Build history of the part. All positions in model axes, mm. Face numbers are marked on the shaded views. A direction names the side the tool comes from. Round coordinates to 2 decimals unless told otherwise and drop trailing zeros. Write each loop counter-clockwise with the first axis right and the second up, starting at its lowest first coordinate (ties: lowest second). Pieces come first, ordered by that corner, then holes. Notation, with made-up numbers: (-36, -4.75) -> (-11, -4.75) arc R32 cw to (-11, 22.25) -> close; hole circle Ø10 at (42.25, 78). An arc over 180 degrees is marked (long way). Answer in a Markdown table with one row per item. Add a question column.
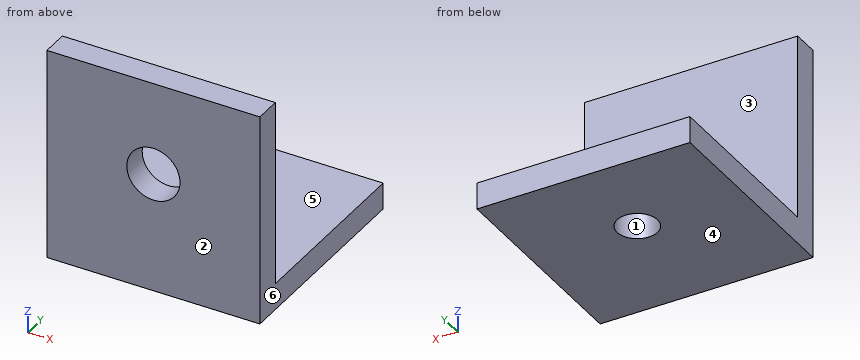
from build123d import *

# Parameters (mm, degrees)
SKETCH1_W           = 25.4
SKETCH1_H           = 25.4
BOSS_EXTRUDE1_DEPTH = 3.175
SKETCH6_W           = 25.4
SKETCH6_H           = 3.175
BOSS_EXTRUDE2_DEPTH = 22.225
SKETCH8_R           = 2.413
CUT_EXTRUDE3_DEPTH  = 3.175
SKETCH9_R           = 3.175
CUT_EXTRUDE4_DEPTH  = 3.175


with BuildPart() as part:
    # Sketch1 → Boss-Extrude1 (new body)
    with BuildSketch(Plane(origin=(0, 0, 0), x_dir=(1, 0, 0), z_dir=(0, 1, 0))):
        Rectangle(SKETCH1_W, SKETCH1_H)
    extrude(amount=BOSS_EXTRUDE1_DEPTH)

    # Sketch6 → Boss-Extrude2 (add)
    with BuildSketch(Plane(origin=(0, 3.175, 0), x_dir=(1, 0, 0), z_dir=(0, 1, 0))):
        with Locations((0, 11.1125)):
            Rectangle(SKETCH6_W, SKETCH6_H)
    extrude(amount=BOSS_EXTRUDE2_DEPTH)

    # Sketch8 → Cut-Extrude3 (cut)
    with BuildSketch(Plane.XY.offset(-9.525)):
        with Locations((0, 14.2875)):
            Circle(SKETCH8_R)
    extrude(amount=-CUT_EXTRUDE3_DEPTH, mode=Mode.SUBTRACT)

    # Sketch9 → Cut-Extrude4 (cut)
    with BuildSketch(Plane(origin=(0, 3.175, 0), x_dir=(1, 0, 0), z_dir=(0, 1, 0))):
        with Locations(Location((0, -1.5875, 0), (0, 0, 270))):
            Circle(SKETCH9_R)
    extrude(amount=-CUT_EXTRUDE4_DEPTH, mode=Mode.SUBTRACT)


solid = part.part
(1) Which spindle directions (+Z, -Z, +X, -X, +Y, -Y) get a long thin tool onto all of the face, cutting with end or side? Do the marked faces 5 and 6. Say none if no direction does.
(2) Probe line 1 along Z through (x, y) = (11, 23.25) (3 decimals); line 2 along Y through (x, z) = (0, -10.6); line 3 along Y through (x, z) = (9, -6.25) (3 decimals). List the from-to ranges inside material, lowest first.
(3) Drop flat-ended pins along their axis: P1, Ø10, axis at x = -2.5, z = -7, coming from the -Y side; P2, Ø6, axis at x = -4.5, z = -2.5, coming from the +Y side (3 decimals). Give the stop position or say it passes through.
(4) Saw through at C-C (z = 7). List the corners of the cut face in (x, y) (3 decimals), plus the area to 3 significant figures.
(5) Saw through at B-B (x = -7.75). List the corners of the cut face in (y, z) (3 decimals), plus the area to 3 significant figures.
(6) Mould opens along Y. For the marked faces 1, 2, 3 and 4 say: pulls with the +Y half, pulls with the -Y half, needs draft (parallel to the pull), parting line crosses it, or undercut.
(7) Saw through at D-D (y = 19). List the corners of the cut face in (x, z) (3 decimals).
(8) Saw through at A-A (x = 0). List the corners of the cut face in (y, z) (1 decimal), plus the area to 3 significant figures.
Answer sheet:
| question | item | result |
|---|---|---|
| 1 | face 5 | +Z, +X, -X, +Y |
| 1 | face 6 | +Z, -Z, +X, +Y, -Y |
| 2 | line 1 | z = -12.7 to -9.525 |
| 2 | line 2 | y = 0 to 11.87, 16.7 to 25.4 |
| 2 | line 3 | y = 0 to 3.175 |
| 3 | P1 | stops at y = 0 |
| 3 | P2 | stops at y = 3.175 |
| 4 | outline | (-12.7, 0) -> (12.7, 0) -> (12.7, 3.175) -> (-12.7, 3.175) -> close |
| 4 | area | 80.6 mm² |
| 5 | outline | (0, -12.7) -> (25.4, -12.7) -> (25.4, -9.525) -> (3.175, -9.525) -> (3.175, 12.7) -> (0, 12.7) -> close |
| 5 | area | 151 mm² |
| 6 | face 1 | undercut |
| 6 | face 2 | pulls with the -Y half |
| 6 | face 3 | pulls with the +Y half |
| 6 | face 4 | needs draft |
| 7 | outline | (-12.7, -12.7) -> (12.7, -12.7) -> (12.7, -9.525) -> (-12.7, -9.525) -> close |
| 8 | outline | (0, -12.7) -> (11.9, -12.7) -> (11.9, -9.5) -> (3.2, -9.5) -> (3.2, -1.6) -> (0, -1.6) -> close; (0, 4.8) -> (3.2, 4.8) -> (3.2, 12.7) -> (0, 12.7) -> close; (16.7, -12.7) -> (25.4, -12.7) -> (25.4, -9.5) -> (16.7, -9.5) -> close |
| 8 | area | 116 mm² |
